Work out the finished part from the listing and answer in its coordinate system (mm). A direction names the side the tool comes from. Give positions to 0.01 mm unless a question says otherwise; leave off trailing zeros. Loops run counter-clockwise (first coordinate to the right, second up) from the corner with the lowest first, then second, coordinate; pieces in that order, holes last. Notation, with made-up numbers: (-20.5, 27.5) - (25.5, 27.5) arc R10 ccw to (25.5, 32.5) - close; hole circle Ø10 at (-4.5, -33.5). An arc over 180 degrees is marked (long way). One line per item, written item: value.
from build123d import *

# Parameters (mm, degrees)
F0_R     = 20.5
F1_DEPTH = 50
F3_DEPTH = 35
F5_W     = 44
F5_H     = 8
F6_DEPTH = 4
F7_R     = 2.5
F9_DEPTH = 2.1


with BuildPart() as f1:
    # F0 (on Top) → F1 (new body)
    with BuildSketch(Plane.XY):
        Circle(F0_R)
    extrude(amount=F1_DEPTH)


with BuildPart() as f3:
    # F2 (on Top) → F3 (new body)
    with BuildSketch(Plane.XY):
        Polygon((-22, 8), (0, 8), (22, 8), (22, 24), (-22, 24), align=None)
    extrude(amount=F3_DEPTH)

    # F4: cut F1
    add(f1.part, mode=Mode.SUBTRACT)

    # F5 (on Top) → F6 (join)
    with BuildSketch(Plane.XY):
        with Locations((0, 28)):
            Rectangle(F5_W, F5_H)
    extrude(amount=F6_DEPTH)

    # F7
    f7_edges = [f3.edges().sort_by_distance(p)[0] for p in [
        (-22, 8, 17.5),
        (22, 8, 17.5),
        (-22, 32, 2),
        (22, 32, 2),
    ]]
    fillet(f7_edges, radius=F7_R)


with BuildPart() as f9:
    # F8 (on Front) → F9 (new body)
    with BuildSketch(Plane.XZ):
        with BuildLine():
            ThreePointArc((0, 13.957158041), (3.7476659403, 15.5094921007), (5.3, 19.257158041))
            ThreePointArc((5.3, 19.257158041), (-3.7476659403, 23.0048239813), (0, 13.957158041))
        make_face()
    extrude(amount=F9_DEPTH)


with BuildPart() as f9_1:
    # F10: moved
    add(f9.part.moved(Location((0, 24, 0))))


with BuildPart() as f3_1:
    add(f3.part)

    # F11: cut F9
    add(f9_1.part, mode=Mode.SUBTRACT)


solid = f3_1.part
1. The mould has two halves that part along Z. Classify faces 3 (the flat face through (0, 21.9, 19)), 4 (the flat face through (0, 23, 0)), 5 (the flat face through (0, 28, 4)), 6 (the cylindrical face through (21.287, 31.248, 2.028)): released by +Z, released by -Z, zero draft, split by the parting line, or undercut.
Output:
face 3: undercut
face 4: released by -Z
face 5: released by +Z
face 6: zero draft
2. Section A-A (y = 18.75) is taken. Write down the section's boundary in (x, z), and give its area (3 significant figures).
Output:
outline: (-22, 0) - (-8.29, 0) - (-8.29, 35) - (-22, 35) - close; (8.29, 0) - (22, 0) - (22, 35) - (8.29, 35) - close
area: 960 mm²
3. Flat-ended cylindrical pins translate along their axes: pin 1 Ø1 at (x, z) = (-15, 24) entering from -Y; pin 2 Ø11.5 at (x, z) = (-2.5, 20) entering from +Y; pin 3 Ø8 at (x, z) = (11, 4.5) entering from -Y. Find the tip coordinate at first contact, or state that the pin passes through.
Output:
pin 1: stops at y = 13.42
pin 2: stops at y = 24
pin 3: stops at y = 13.97
4. For faces 1 (the cylindrical face through (-21.287, 31.248, 2.028)), 2 (the flat face through (5, 24, 23)), determine the directions among +Z, -Z, +X, -X, +Y, -Y from which every point of the face is accessible in a straight line to the end or side of a thin tool.
Output:
face 1: +Z, -Z, -X, +Y
face 2: +Z, +X, -X, +Y
5. Section D-D (y = 26) is taken. Write down the section's boundary in (x, z).
Output:
outline: (-22, 0) - (22, 0) - (22, 4) - (-22, 4) - close
6. Find the intervals of material crossed by line 1 along Z through (x, y) = (0, 23.25); line 2 along Y through (x, z) = (19, 23); line 3 along Z through (x, y) = (-1.5, 26.5), in increasing order.
Output:
line 1: z = 0 to 13.96, 24.56 to 35
line 2: y = 8 to 24
line 3: z = 0 to 4
7. Section B-B (z = 21) is taken. Write down the section's boundary in (x, y).
Output:
outline: (-22, 10.5) arc R2.5 ccw to (-19.5, 8) - (-18.87, 8) arc R20.5 cw to (18.87, 8) - (19.5, 8) arc R2.5 ccw to (22, 10.5) - (22, 24) - (5.01, 24) - (5.01, 21.9) - (-5.01, 21.9) - (-5.01, 24) - (-22, 24) - close
8. Section C-C (x = -9) is taken. Write down the section's boundary in (y, z), and give its area (3 significant figures).
Output:
outline: (18.42, 0) - (32, 0) - (32, 4) - (24, 4) - (24, 35) - (18.42, 35) - close
area: 227 mm²
